Build history of the part. All positions in model axes, mm. A direction names the side the tool comes from. Coordinates: 2 decimals unless noted, no trailing zeros. Loops run counter-clockwise (first coordinate to the right, second up) from the corner with the lowest first, then second, coordinate; pieces in that order, holes last.
(1) Slice it at B-B (y = -1.5). Give the cut face in (x, z).
(2) Two-plate mould, pull along Y, no slides. Class faces 4 (the face through (15, -22.5, 3)), 5 (the face through (0, 12.5, 6)), 6 (the face through (-25, 0, 6)), 7 (the face through (0, 0, 10.5)): pulls with the +Y half, pulls with the -Y half, needs draft (parallel to the pull), parting line crosses it, or undercut.
(3) Wall check: L1, parallel to X at y = -14, z = 5.75; L2, parallel to X at y = -4, z = 7.5; L3, parallel to Z at x = -21, y = 4. Give the ranges that are in metal, low to high.
(4) Slice it at D-D (x = 18). Give the cut face in (y, z), and give its area (3 significant figures).
(5) Tool access for faces 1 (the face through (0, -11, 6)), 2 (the face through (0, 0, 0)), 3 (the face through (12.95, -16.67, 7.68)): list every direction of +Z, -Z, +X, -X, +Y, -Y with a clear straight run to the whole face (end or side of a thin tool).
(6) Slice it at C-C (y = -18). Give the cut face in (x, z), and give its area (3 significant figures).
(7) Flat gauge pins, fed straight in: P1, Ø2, axis at x = -3, z = 1.5, coming from the -Y side; P2, Ø2, axis at y = -15.5, z = 3, coming from the -X side; P3, Ø4, axis at x = -14.83, z = 5.95, coming from the -Y side. Where does each tip first touch, or does it go through?
(8) Slice it at A-A (x = 5.5). Give the cut face in (y, z).
from build123d import *

# Parameters (mm, degrees)
F0_W     = 50
F0_H     = 25
F1_DEPTH = 12
F2_R     = 4.0545181675
F3_DEPTH = 10
F4_T     = -1.5
F5_R     = 4.327746069
F6_DEPTH = 3
F8_R     = 1
F9_DEPTH = 20


# Not quite as in the source:
# - a fillet or chamfer that OpenCascade refuses, or shapes differently, is made with other operations: its cross-section is extruded or revolved along the edge and cut away or added


with BuildPart() as f1:
    # F0 (on Top) → F1 (new body)
    with BuildSketch(Plane.XY):
        Rectangle(F0_W, F0_H)
    extrude(amount=F1_DEPTH)

    # F2 (on face) → F3 (join)
    with BuildSketch(Plane.XZ.offset(12.5)):
        with Locations((-14.8313278332, 5.9491097927)):
            Circle(F2_R)
        with Locations((14.8313278332, 5.9491097927)):
            Circle(F2_R)
    extrude(amount=F3_DEPTH)

    # F4
    f4_openings = [f1.faces().sort_by_distance(p)[0] for p in [
        (14.831328, -22.5, 5.94911),
        (-14.831328, -22.5, 5.94911),
    ]]
    offset(amount=F4_T, openings=f4_openings, kind=Kind.INTERSECTION)

    # F5 (on face) → F6 (join)
    with BuildSketch(Plane.XZ.offset(22.5)):
        with Locations((-14.8313278332, 5.9491097927)):
            Circle(F5_R)
    extrude(amount=-F6_DEPTH)

    # F7: fillet of radius 3 on 1 edges, made by hand

    # F7_s1 → F7_t2 (revolve, cut)
    with BuildSketch(Plane.XY.offset(5.9491097927)):
        with BuildLine():
            ThreePointArc((-10.7768096658, -19.5), (-10.5726846068, -20.1106963365), (-10.5035817643, -20.7508852557))
            Line((-10.5035817643, -20.7508852557), (-10.5035817643, -19.5))
            Line((-10.5035817643, -19.5), (-10.7768096658, -19.5))
        make_face()
    revolve(axis=Axis((-14.8313278332, -19.5, 5.9491097927), (0, -1, 0)), mode=Mode.SUBTRACT)

    # F8
    f8_edges = [f1.edges().sort_by_distance(p)[0] for p in [
        (-19.159074, -22.5, 5.94911),
    ]]
    fillet(f8_edges, radius=F8_R)

    # F9 (cut): a face of the model
    f9_faces = [f1.faces().sort_by_distance(p)[0] for p in [
        (-14.8313278332, -22.5, 5.9491097927),
    ]]
    extrude(f9_faces, amount=-F9_DEPTH, mode=Mode.SUBTRACT)


solid = f1.part
Response values:
1. outline: (-25, 0) - (25, 0) - (25, 12) - (-25, 12) - close; hole (-23.5, 1.5) - (23.5, 1.5) - (23.5, 10.5) - (-23.5, 10.5) - close
2. face 4: pulls with the -Y half
2. face 5: pulls with the +Y half
2. face 6: needs draft
2. face 7: undercut
3. L1: x = -18.88 to -18.15, -11.51 to -10.78, 10.78 to 12.28, 17.38 to 18.88
3. L2: x = -25 to -23.5, 23.5 to 25
3. L3: z = 0 to 1.5, 10.5 to 12
4. outline: (-22.5, 3.42) - (-12.5, 3.42) - (-12.5, 0) - (12.5, 0) - (12.5, 12) - (-12.5, 12) - (-12.5, 8.48) - (-22.5, 8.48) - close; hole (-11, 1.5) - (11, 1.5) - (11, 10.5) - (-11, 10.5) - close
4. area: 153 mm2
5. face 1: none
5. face 2: -Z, +X, -X, +Y, -Y
5. face 3: -Y
6. outline: circle Ø8.11 at (-14.83, 5.95); circle Ø8.11 at (14.83, 5.95); hole circle Ø6.66 at (-14.83, 5.95); hole circle Ø5.11 at (14.83, 5.95)
6. area: 48.0 mm2
7. P1: stops at y = -12.5
7. P2: stops at x = -18.39
7. P3: stops at y = 11
8. outline: (-12.5, 0) - (12.5, 0) - (12.5, 12) - (-12.5, 12) - close; hole (-11, 1.5) - (11, 1.5) - (11, 10.5) - (-11, 10.5) - close
